```python
from build123d import *

# Parameters (mm, degrees)
SKETCH_1_W          = 87
SKETCH_1_H          = 85.2
EXTRUDE_1_DEPTH     = 4
SKETCH_2_W          = 60
SKETCH_2_H          = 11
CUT_EXTRUDE_1_DEPTH = 4
SKETCH_3_R          = 1.75
CUT_EXTRUDE_2_DEPTH = 4
SKETCH_4_R          = 1.6
CUT_EXTRUDE_3_DEPTH = 4
FILLET_3_R          = 2


with BuildPart() as part:
    # 草图1 → 凸台-拉伸1 (new body)
    with BuildSketch(Plane(origin=(0, 0, 0), x_dir=(1, 0, 0), z_dir=(0, 1, 0))):
        Rectangle(SKETCH_1_W, SKETCH_1_H)
    extrude(amount=EXTRUDE_1_DEPTH)

    # 草图2 → 切除-拉伸1 (cut)
    with BuildSketch(Plane(origin=(0, 4, 0), x_dir=(1, 0, 0), z_dir=(0, 1, 0))):
        with Locations((-43.5, 42.6)):
            Rectangle(SKETCH_2_W, SKETCH_2_H)
        with Locations((43.5, 42.6)):
            Rectangle(SKETCH_2_W, SKETCH_2_H)
        with Locations((43.5, -42.6)):
            Rectangle(SKETCH_2_W, SKETCH_2_H)
        with Locations((-43.5, -42.6)):
            Rectangle(SKETCH_2_W, SKETCH_2_H)
    extrude(amount=-CUT_EXTRUDE_1_DEPTH, mode=Mode.SUBTRACT)

    # 草图3 → 切除-拉伸2 (cut)
    with BuildSketch(Plane(origin=(0, 4, 0), x_dir=(1, 0, 0), z_dir=(0, 1, 0))):
        with Locations(Location((-32, 16, 0), (0, 0, 270))):
            Circle(SKETCH_3_R)
        with Locations(Location((32, 16, 0), (0, 0, 270))):
            Circle(SKETCH_3_R)
        with Locations(Location((-32, -16, 0), (0, 0, 270))):
            Circle(SKETCH_3_R)
        with Locations(Location((32, -16, 0), (0, 0, 270))):
            Circle(SKETCH_3_R)
    extrude(amount=-CUT_EXTRUDE_2_DEPTH, mode=Mode.SUBTRACT)

    # 草图4 → 切除-拉伸3 (cut)
    with BuildSketch(Plane(origin=(0, 4, 0), x_dir=(1, 0, 0), z_dir=(0, 1, 0))):
        with Locations(Location((-8, 39.85, 0), (0, 0, 270))):
            Circle(SKETCH_4_R)
        with Locations(Location((8, 39.85, 0), (0, 0, 270))):
            Circle(SKETCH_4_R)
        with Locations(Location((8, -39.85, 0), (0, 0, 90))):
            Circle(SKETCH_4_R)
        with Locations(Location((-8, -39.85, 0), (0, 0, 90))):
            Circle(SKETCH_4_R)
    extrude(amount=-CUT_EXTRUDE_3_DEPTH, mode=Mode.SUBTRACT)

    # 圆角3
    fillet_3_edges = [part.edges().sort_by_distance(p)[0] for p in [
        (-13.5, 2, -42.6),
        (-43.5, 2, -37.1),
        (-13.5, 2, -37.1),
        (43.5, 2, -37.1),
        (13.5, 2, -42.6),
        (13.5, 2, -37.1),
        (43.5, 2, 37.1),
        (13.5, 2, 37.1),
        (13.5, 2, 42.6),
        (-43.5, 2, 37.1),
        (-13.5, 2, 42.6),
        (-13.5, 2, 37.1),
    ]]
    fillet(fillet_3_edges, radius=FILLET_3_R)


solid = part.part
```
CAD build for the part. Positions are in the model's coordinates, mm. A direction names the side the tool comes from. Give positions to 0.01 mm unless a question says otherwise; leave off trailing zeros. Loops run counter-clockwise (first coordinate to the right, second up) from the corner with the lowest first, then second, coordinate; pieces in that order, holes last. Notation, with made-up numbers: M 77,69 L 131,69 A16 cw 131,80 Z; hole C 63,24.25 d6. An arc over 180 degrees is marked long. Use one line per item in the form item = value.
Item 1: Two-plate mould, pull along X, no slides. Class faces 4 (the face through (0, 2, -42.6)), 5 (the face through (-14.1, 1.97, -37.67)), 6 (the face through (9, 2, 41.1)): pulls with the +X half, pulls with the -X half, needs draft (parallel to the pull), parting line crosses it, or undercut.
Determined:
face_4 = needs draft
face_5 = pulls with the -X half
face_6 = undercut
Item 2: Flat gauge pins, fed straight in: pin 1 (6 mm diameter, centred on x = 4, z = -7.5, fed in from -Y); pin 2 (0.8 mm diameter, centred on y = 3, z = -40, fed in from +X); pin 3 (1.5 mm diameter, centred on x = -16.5, y = 3.5, fed in from +Z); pin 4 (2 mm diameter, centred on x = 30, y = 1.5, fed in from -Z). Where does each tip first touch, or does it go through?
Determined:
pin_1 = 0
pin_2 = 13.5
pin_3 = 37.1
pin_4 = -37.1
Item 3: Which spindle directions (+Z, -Z, +X, -X, +Y, -Y) get a long thin tool onto all of the face, cutting with end or side? Do faces 1 (the face through (-29, 2, -37.1)), 2 (the face through (-29, 2, 37.1)), 3 (the face through (14.07, 1.97, -37.7)). Say none if no direction does.
Determined:
face_1 = -Z, -X, +Y, -Y
face_2 = +Z, -X, +Y, -Y
face_3 = -Z, +X, +Y, -Y
Item 4: Slice it at C-C (y = 0.9). Count the separate pieces of the cut face and the enclosed holes in it, plus the area to 3 significant figures.
Determined:
separate_pieces = 1
enclosed_holes = 8
area = 6,680 mm2
Item 5: Drill centre lines: probe 1 along X at (y, z) = (2.05, 39.85); probe 2 along X at (y, z) = (1, 16); probe 3 along Z at (x, y) = (16, 2.1). Where is each one in solid material? Low to high. Write a range as from..to.
Determined:
probe_1 = -13.5..-9.6, -6.4..6.4, 9.6..13.5
probe_2 = -43.5..-33.75, -30.25..30.25, 33.75..43.5
probe_3 = -37.1..37.1
Item 6: Slice it at D-D (x = 37.5). List the corners of the cut face in (y, z).
Determined:
outline = M 0,-37.1 L 4,-37.1 L 4,37.1 L 0,37.1 Z
Item 7: Slice it at B-B (z = -16). List the corners of the cut face in (x, y), plus the area to 3 significant figures.
Determined:
outline = M -43.5,0 L -33.75,0 L -33.75,4 L -43.5,4 Z; M -30.25,0 L 30.25,0 L 30.25,4 L -30.25,4 Z; M 33.75,0 L 43.5,0 L 43.5,4 L 33.75,4 Z
area = 320 mm2
Item 8: Slice it at A-A (x = -32). List the corners of the cut face in (y, z).
Determined:
outline = M 0,-37.1 L 4,-37.1 L 4,-17.75 L 0,-17.75 Z; M 0,-14.25 L 4,-14.25 L 4,14.25 L 0,14.25 Z; M 0,17.75 L 4,17.75 L 4,37.1 L 0,37.1 Z
